```python
from build123d import *

# Parameters (mm, degrees)
F1_DEPTH = 50.8
F2_T     = -6.35
F3_R     = 6.35
F4_R     = 20.639799
F5_DEPTH = 25.4


with BuildPart() as f1:
    # F0 (on Front) → F1 (new body)
    with BuildSketch(Plane.XZ):
        Polygon((-46.398684, 47.853038), (-46.398684, -36.724649), (36.554363, -36.724649), (37.55359, 47.853038), align=None)
    extrude(amount=-F1_DEPTH)

    # F2
    f2_openings = [f1.faces().sort_by_distance(p)[0] for p in [
        (-4.671856, 0, 5.648586),
    ]]
    offset(amount=F2_T, openings=f2_openings)

    # F3
    f3_edges = [f1.edges().sort_by_distance(p)[0] for p in [
        (37.55359, 25.4, 47.853038),
        (-46.398684, 25.4, 47.853038),
        (36.554363, 25.4, -36.724649),
        (-46.398684, 25.4, -36.724649),
    ]]
    fillet(f3_edges, radius=F3_R)

    # F4 (on face) → F5 (join)
    with BuildSketch(Plane(origin=(0, 50.8, 0), x_dir=(-1, 0, 0), z_dir=(0, 1, 0))):
        with Locations((4.460279, 5.489179)):
            Circle(F4_R)
    extrude(amount=F5_DEPTH)


solid = f1.part
```
Model file for the job. Use its own axes, mm. A direction names the side the tool comes from. Coordinates: 2 decimals unless noted, no trailing zeros. Loops run counter-clockwise (first coordinate to the right, second up) from the corner with the lowest first, then second, coordinate; pieces in that order, holes last. Notation, with made-up numbers: (58, 11.25) -> (100, 11.25) arc R9 ccw to (100, 22.25) -> close; hole circle Ø11 at (-24.75, 49.5). An arc over 180 degrees is marked (long way). Answer as a JSON object with one key per item and string values.
Q1. Pull direction X, two halves, no side cores. Call faces 1 (the flat face through (-5, 25, -36.725)), 2 (the flat face through (-5, 22, -30.375)), 3 (the cylindrical face through (34.69, 25.76, -34.94)): released by +X, released by -X, zero draft, split by the parting line, or undercut.
Report:
{"face 1": "zero draft", "face 2": "undercut", "face 3": "released by +X"}
Q2. Cut at C-C (z = -27). List the corners of the cut face in (x, y), and give its area (3 significant figures).
Report:
{"outline": "(-46.4, 0) -> (-40.05, 0) -> (-40.05, 44.45) -> (30.32, 44.45) -> (30.32, 0) -> (36.67, 0) -> (36.67, 50.8) -> (-46.4, 50.8) -> close", "area": "1,090 mm2"}
Q3. Cut at D-D (x = 15). List the corners of the cut face in (y, z), and give its area (3 significant figures).
Report:
{"outline": "(0, -36.72) -> (50.8, -36.72) -> (50.8, -1.39) -> (76.2, -1.39) -> (76.2, 12.37) -> (50.8, 12.37) -> (50.8, 47.85) -> (0, 47.85) -> (0, 41.5) -> (44.45, 41.5) -> (44.45, -30.37) -> (0, -30.37) -> close", "area": "1,450 mm2"}
Q4. Cut at B-B (x = 25). List the corners of the cut face in (y, z).
Report:
{"outline": "(0, -36.72) -> (50.8, -36.72) -> (50.8, 47.85) -> (0, 47.85) -> (0, 41.5) -> (44.45, 41.5) -> (44.45, -30.37) -> (0, -30.37) -> close"}
Q5. Cut at A-A (y = 15). List the corners of the cut face in (x, z).
Report:
{"outline": "(-46.4, -30.37) arc R6.35 ccw to (-40.05, -36.72) -> (30.28, -36.72) arc R6.35 ccw to (36.63, -30.45) -> (37.48, 41.43) arc R6.35 ccw to (31.13, 47.85) -> (-40.05, 47.85) arc R6.35 ccw to (-46.4, 41.5) -> close; hole (-40.05, -30.37) -> (30.28, -30.37) -> (31.13, 41.5) -> (-40.05, 41.5) -> close"}
Q6. 3-axis set-ups, long thin cutter, end or side, ignore diameter. For faces 4 (the flat face through (-24, 50.8, 16)), 5 (the flat face through (-4, 76.2, 6)), 6 (the flat face through (-4, 22, 41.503)): which of +Z, -Z, +X, -X, +Y, -Y reach the whole face in a straight line?
Report:
{"face 4": "+Y", "face 5": "+Z, -Z, +X, -X, +Y", "face 6": "-Y"}
Q7. Probe probe 1 along Z at (x, y) = (-29, 17.5); probe 2 along X at (y, z) = (25, -8); probe 3 along X at (y, z) = (22, 21). List the from-to ranges inside material, lowest first.
Report:
{"probe 1": "z = -36.72 to -30.37, 41.5 to 47.85", "probe 2": "x = -46.4 to -40.05, 30.54 to 36.89", "probe 3": "x = -46.4 to -40.05, 30.89 to 37.24"}
Q8. Flat gauge pins, fed straight in: P1, Ø1, axis at x = 20, z = 3, coming from the -Y side; P2, Ø8, axis at x = 4.5, y = 68.5, coming from the -Z side; P3, Ø10, axis at y = 12, z = 23.5, coming from the +X side. Where does each tip first touch, or does it go through?
Report:
{"P1": "stops at y = 44.45", "P2": "stops at z = -14.55", "P3": "stops at x = 37.32"}
